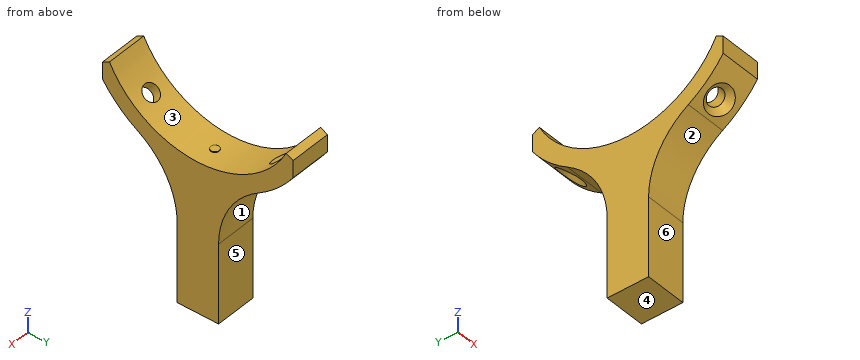
```python
from build123d import *

# Parameters (mm, degrees)
F1_DEPTH       = 5
F5_D           = 2
F5_DEPTH       = 5
F5_CSINK_D     = 3.5
F5_CSINK_ANGLE = 90
F8_D           = 2
F8_DEPTH       = 5
F8_CSINK_D     = 3.5
F8_CSINK_ANGLE = 90
F10_R          = 0.5
F11_DEPTH      = 0.1


with BuildPart() as f1:
    # F0 (on Right) → F1 (new body)
    with BuildSketch(Plane.YZ):
        with BuildLine():
            ThreePointArc((2.5, -20.487801), (3.779813, -15.593076), (7.291667, -11.951217))
            ThreePointArc((7.291667, -11.951217), (9.602899, -10.187459), (11.5, -7.98436))
            Line((11.5, -7.98436), (11.5, -5.930411))
            Line((11.5, -5.930411), (10.665365, -5.5))
            ThreePointArc((10.665365, -5.5), (0, -12), (-10.665365, -5.5))
            Line((-10.665365, -5.5), (-11.5, -5.930411))
            Line((-11.5, -5.930411), (-11.5, -7.98436))
            ThreePointArc((-11.5, -7.98436), (-9.602899, -10.187459), (-7.291667, -11.951217))
            ThreePointArc((-7.291667, -11.951217), (-3.779813, -15.593076), (-2.5, -20.487801))
            Line((-2.5, -20.487801), (-2.5, -30))
            Line((-2.5, -30), (2.5, -30))
            Line((2.5, -30), (2.5, -20.487801))
        make_face()
    extrude(amount=F1_DEPTH)

    # F5
    with Locations(Plane(origin=(0, 8.999027, -10.724622), x_dir=(1, 0, 0), z_dir=(0, 0.642788, -0.766044))):
        with Locations((2.5, 0)):
            CounterSinkHole(F5_D / 2, F5_CSINK_D / 2, depth=F5_DEPTH, counter_sink_angle=F5_CSINK_ANGLE)

    # F8
    with Locations(Plane(origin=(0, -8.999027, -10.724622), x_dir=(1, 0, 0), z_dir=(0, -0.642788, -0.766044))):
        with Locations((2.5, 0)):
            CounterSinkHole(F8_D / 2, F8_CSINK_D / 2, depth=F8_DEPTH, counter_sink_angle=F8_CSINK_ANGLE)

    # F10 (on offset) → F11 (join)
    with BuildSketch(Plane.XY.offset(-12)):
        with Locations((2.5, 0)):
            Circle(F10_R)
    extrude(amount=F11_DEPTH)


solid = f1.part
```
Work out the finished part from the listing and answer in its coordinate system (mm). Face numbers are marked on the shaded views. A direction names the side the tool comes from. Give positions to 0.01 mm unless a question says otherwise; leave off trailing zeros. Order: outer loops, then holes, each group sorted by start corner. A loop starts at its lowest first (then second) coordinate and runs counter-clockwise, first axis right, second up.
1. The mould has two halves that part along Y. Classify the marked faces 1, 2 and 3: released by +Y, released by -Y, zero draft, split by the parting line, or undercut.
Result sheet:
face 1: released by +Y
face 2: released by -Y
face 3: undercut
2. Section C-C, the plane z = -25.75 is taken. Determine the outline of the cut face in (x, y).
Result sheet:
outline: (0, -2.5) - (5, -2.5) - (5, 2.5) - (0, 2.5) - close
3. Section D-D, the plane z = -15 is taken. Determine the outline of the cut face in (x, y), and give its area (3 significant figures).
Result sheet:
outline: (0, -4.14) - (5, -4.14) - (5, 4.14) - (0, 4.14) - close
area: 41.4 mm2
4. Each of these flat-tipped pins is pushed along its axis until it touches: P1, Ø1.5, axis at x = 0.5, y = 5.5, coming from the -Z side; P2, Ø1.1, axis at x = 2.5, y = 0, coming from the +Z side; P3, Ø1.5, axis at x = 1.5, z = -24, coming from the -Y side. Where does it stop, or does it pass through?
Result sheet:
P1: stops at z = -14.17
P2: stops at z = -11.9
P3: stops at y = -2.5
5. Section B-B, the plane x = 2.5 is taken. Determine the outline of the cut face in (y, z).
Result sheet:
outline: (-11.5, -7.98) arc R14 ccw to (-10.2, -9.59) - (-9.28, -9.51) - (-8.45, -8.52) arc R12 cw to (-10.67, -5.5) - (-11.5, -5.93) - close; (-7.75, -10.79) - (-7.67, -11.71) arc R14 ccw to (-7.29, -11.95) arc R10 cw to (-2.5, -20.49) - (-2.5, -30) - (2.5, -30) - (2.5, -20.49) arc R10 cw to (7.29, -11.95) arc R14 ccw to (7.67, -11.71) - (7.75, -10.79) - (6.92, -9.8) arc R12 cw to (0.5, -11.99) - (0.5, -11.9) - (-0.5, -11.9) - (-0.5, -11.99) arc R12 cw to (-6.92, -9.8) - close; (8.45, -8.52) - (9.28, -9.51) - (10.2, -9.59) arc R14 ccw to (11.5, -7.98) - (11.5, -5.93) - (10.67, -5.5) arc R12 cw to start
6. Straight lines are drawn through the part: L1, parallel to Y at x = 3.35, z = -27; L2, parallel to Y at x = 3.7, z = -8.75; L3, parallel to Y at x = 1.85, z = -10.25. For each, find the intervals that lie inside material, in ascending order.
Result sheet:
L1: y = -2.5 to 2.5
L2: y = -10.93 to -8.21, 8.21 to 10.93
L3: y = -7.61 to -6.24, 6.24 to 7.61
7. Section A-A, the plane y = 0 is taken. Determine the outline of the cut face in (x, z).
Result sheet:
outline: (0, -30) - (5, -30) - (5, -12) - (3, -12) - (3, -11.9) - (2, -11.9) - (2, -12) - (0, -12) - close
8. For the marked faces 4, 5 and 6, determine the directions among +Z, -Z, +X, -X, +Y, -Y from which every point of the face is accessible in a straight line to the end or side of a thin tool.
Result sheet:
face 4: -Z, +X, -X, +Y, -Y
face 5: -Z, +X, -X, +Y
face 6: -Z, +X, -X, -Y
